Part model, mm, in its own coordinate system. A direction names the side the tool comes from. Round coordinates to 2 decimals unless told otherwise and drop trailing zeros. Write each loop counter-clockwise with the first axis right and the second up, starting at its lowest first coordinate (ties: lowest second). Pieces come first, ordered by that corner, then holes.
```python
from build123d import *

# Parameters (mm, degrees)
SKETCH_1_R               = 1.55
EXTRUDE_1_DEPTH          = 1.5
SKETCH_2_R               = 0.6
CUT_EXTRUDE_1_DEPTH      = 1
CUT_EXTRUDE_1_DEPTH_BACK = 4
FILLET_1_R               = 1
CUT_EXTRUDE_2_DEPTH      = 4
FILLET_2_R               = 0.6


with BuildPart() as part:
    # 草图1 → 凸台-拉伸1 (new body, symmetric)
    with BuildSketch(Plane.XY):
        Polygon((-20.5, 3.5), (-10.025, 3.5), (-10.025, 6), (10.025, 6), (10.025, 3.5), (20.5, 3.5), (20.5, -3.5), (10.025, -3.5), (10.025, -6), (-10.025, -6), (-10.025, -3.5), (-20.5, -3.5), align=None)
        with Locations((-17, 0)):
            Circle(SKETCH_1_R, mode=Mode.SUBTRACT)
        with Locations((-6, 0)):
            Circle(SKETCH_1_R, mode=Mode.SUBTRACT)
        with Locations((6, 0)):
            Circle(SKETCH_1_R, mode=Mode.SUBTRACT)
        with Locations((17, 0)):
            Circle(SKETCH_1_R, mode=Mode.SUBTRACT)
    extrude(amount=EXTRUDE_1_DEPTH, both=True)

    # 草图2 → 切除-拉伸1 (cut, two sides)
    with BuildSketch(Plane.XY.offset(1.5)) as cut_extrude_1_sk:
        with Locations((-10.025, 4.1)):
            Circle(SKETCH_2_R)
        with Locations((-10.025, -4.1)):
            Circle(SKETCH_2_R)
        with Locations((10.025, 4.1)):
            Circle(SKETCH_2_R)
        with Locations((10.025, -4.1)):
            Circle(SKETCH_2_R)
    extrude(amount=CUT_EXTRUDE_1_DEPTH, mode=Mode.SUBTRACT)
    extrude(cut_extrude_1_sk.sketch, amount=-CUT_EXTRUDE_1_DEPTH_BACK, mode=Mode.SUBTRACT)

    # 圆角1
    fillet_1_edges = [part.edges().sort_by_distance(p)[0] for p in [
        (20.5, -3.5, 0),
        (20.5, 3.5, 0),
        (-20.5, -3.5, 0),
        (-20.5, 3.5, 0),
    ]]
    fillet(fillet_1_edges, radius=FILLET_1_R)

    # 草图4 → 切除-拉伸2 (cut, through all)
    with BuildSketch(Plane.XY.offset(1.5)):
        with BuildLine():
            Line((-13.782469891, 1.5), (-9.217530109, 1.5))
            ThreePointArc((-9.217530109, 1.5), (-9.55, 0), (-9.217530109, -1.5))
            Line((-9.217530109, -1.5), (-13.782469891, -1.5))
            ThreePointArc((-13.782469891, -1.5), (-13.45, 0), (-13.782469891, 1.5))
        make_face()
        with BuildLine():
            Line((-5.406282896, 3.5), (5.406282896, 3.5))
            ThreePointArc((5.406282896, 3.5), (2.45, 0), (5.406282896, -3.5))
            Line((5.406282896, -3.5), (-5.406282896, -3.5))
            ThreePointArc((-5.406282896, -3.5), (-2.45, 0), (-5.406282896, 3.5))
        make_face()
        with BuildLine():
            Line((13.782469891, 1.5), (9.217530109, 1.5))
            ThreePointArc((9.217530109, 1.5), (9.55, 0), (9.217530109, -1.5))
            Line((9.217530109, -1.5), (13.782469891, -1.5))
            ThreePointArc((13.782469891, -1.5), (13.45, 0), (13.782469891, 1.5))
        make_face()
    extrude(amount=-CUT_EXTRUDE_2_DEPTH, mode=Mode.SUBTRACT)

    # 圆角2
    fillet_2_edges = [part.edges().sort_by_distance(p)[0] for p in [
        (-13.782469891, -1.5, 0),
        (-13.782469891, 1.5, 0),
        (-9.217530109, 1.5, 0),
        (-9.217530109, -1.5, 0),
        (-5.406282896, -3.5, 0),
        (-5.406282896, 3.5, 0),
        (5.406282896, 3.5, 0),
        (5.406282896, -3.5, 0),
        (13.782469891, 1.5, 0),
        (13.782469891, -1.5, 0),
        (9.217530109, -1.5, 0),
        (9.217530109, 1.5, 0),
    ]]
    fillet(fillet_2_edges, radius=FILLET_2_R)


solid = part.part
```
Q1. Mould opens along Y. For faces 4 (the flat face through (-15, -3.5, 0)), 5 (the flat face through (0, 4, 1.5)), 6 (the cylindrical face through (4.45, 0.07, -0.02)) say: +Y half, -Y half, draft (parallel to the pull), parting line (faces both ways), or undercut.
Values follow:
face 4: -Y half
face 5: draft
face 6: undercut
Q2. Drop flat-ended pins along their axis: pin 1 (0.9 mm diameter, centred on x = 17, z = 0, fed in from +Y); pin 2 (1 mm diameter, centred on y = -5.5, z = 0, fed in from -X) (3 decimals); pin 3 (1.4 mm diameter, centred on x = -11, z = -0.5, fed in from -Y). Give the stop position or say it passes through.
Values follow:
pin 1: stops at y = 3.5
pin 2: stops at x = -10.025
pin 3: stops at y = -3.5
Q3. Cut at A-A on x = 17. Write the cut outline in (y, z), plus the area to 3 significant figures.
Values follow:
outline: (-3.5, -1.5) - (-1.55, -1.5) - (-1.55, 1.5) - (-3.5, 1.5) - close; (1.55, -1.5) - (3.5, -1.5) - (3.5, 1.5) - (1.55, 1.5) - close
area: 11.7 mm2
Q4. Cut at D-D on x = -10.5. Write the cut outline in (y, z).
Values follow:
outline: (-3.5, -1.5) - (-1.5, -1.5) - (-1.5, 1.5) - (-3.5, 1.5) - close; (1.5, -1.5) - (3.5, -1.5) - (3.5, 1.5) - (1.5, 1.5) - close
Q5. Which spindle directions (+Z, -Z, +X, -X, +Y, -Y) get a long thin tool onto all of the face, cutting with end or side? Do faces 1 (the flat face through (-20.5, 0, 0)), 2 (the cylindrical face through (-2.45, -0.04, 0.02)), 3 (the flat face through (-10.025, 5, 0)). Say none if no direction does.
Values follow:
face 1: +Z, -Z, -X, +Y, -Y
face 2: +Z, -Z
face 3: +Z, -Z, -X, +Y
Q6. Cut at B-B on y = 0. State how many separate pieces and enclosed holes the cut face has, plus the area to 3 significant figures.
Values follow:
separate pieces: 8
enclosed holes: 0
area: 47.7 mm2
Q7. Wall check: L1, parallel to Y at x = 6, z = -0.55; L2, parallel to Y at x = -17, z = 0.8; L3, parallel to Y at x = -3.5, z = -0.1. Give the ranges that are in metal, low to high.
Values follow:
L1: y = -6 to -1.55, 1.55 to 6
L2: y = -3.5 to -1.55, 1.55 to 3.5
L3: y = -6 to -3.27, -2.53 to 2.53, 3.27 to 6
